Input: dimensioned drawing with shaded views. Units: mm. Origin: part minimum x, y, z. A direction names the side the tool comes from. Round coordinates to 2 decimals unless told otherwise and drop trailing zeros. Order: outer loops, then holes, each group sorted by start corner. A loop starts at its lowest first (then second) coordinate and runs counter-clockwise, first axis right, second up. Notation, with made-up numbers: (87.5, -25) - (135.5, -25) arc R18 cw to (135.5, -21) - close; hole circle Ø9 at (-9.75, 12). An arc over 180 degrees is marked (long way). Put each result on its own line as item: value. Start each with the question number.
(1) Section A-A (x = 90). Output: boundary loops of the cut face in (y, z) (1 decimal), and give its area (3 significant figures).
(2) Pull-direction query (X, two-part tool) for the marked faces 1, 2, 3 and 4; classes: released by +X, released by -X, zero draft, split by the parting line, or undercut.
(3) Section B-B (y = 33.5). Output: boundary loops of the cut face in (x, z), and give its area (3 significant figures).
(4) Material intervals for L1, parallel to X at y = 68, z = 3.5; L2, parallel to X at y = 10.5, z = 40; L3, parallel to Y at x = 12.7, z = 2 (1 decimal), sorted ascending. Write a range as [from, to].
(5) Access query for the marked faces 5, 6, 7 and 8. Directions: +Z, -Z, +X, -X, +Y, -Y. A direction counts if a zero-diameter tool reaches every point of the face in a straight line with its end or side. Return the directions, or none.
(6) Section D-D (z = 18.5). Output: boundary loops of the cut face in (x, y) (1 decimal), and give its area (3 significant figures).
(7) Section C-C (x = 12.7). Output: boundary loops of the cut face in (y, z) (1 decimal).
(8) Pin query (flat end, axial travel): P1, Ø20.5, axis at x = 95, z = 10, coming from the +Y side; P2, Ø8.5, axis at x = 50.8, y = 83.92, coming from the +Z side; P3, Ø3, axis at x = 35.5, z = 8.5, coming from the +Y side; P4, Ø20.5, axis at x = 51, y = 15.5, coming from the +Z side. Return the tip coordinate at first contact, or that it passes through.
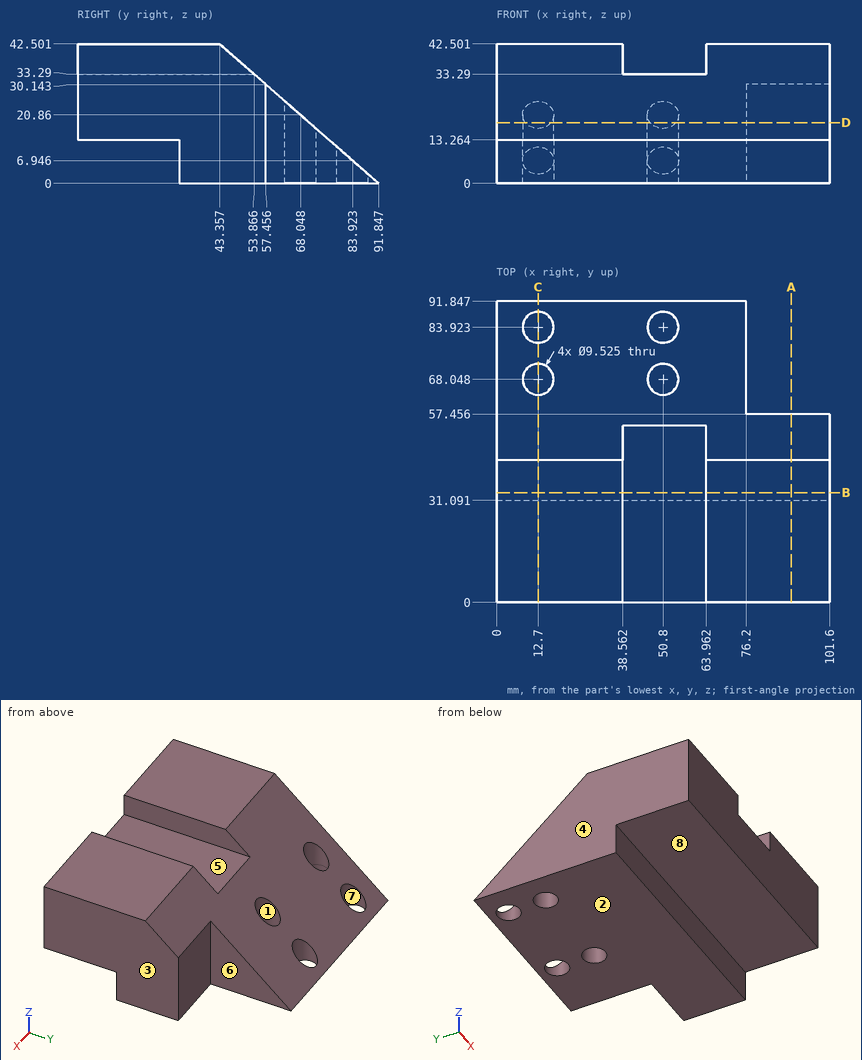
Checks:
1. outline: (0, 13.3) - (31.1, 13.3) - (31.1, 0) - (57.5, 0) - (57.5, 30.1) - (43.4, 42.5) - (0, 42.5) - close
1. area: 1,940 mm²
2. face 1: undercut
2. face 2: zero draft
2. face 3: released by +X
2. face 4: released by -X
3. outline: (0, 0) - (101.6, 0) - (101.6, 42.5) - (63.96, 42.5) - (63.96, 33.29) - (38.56, 33.29) - (38.56, 42.5) - (0, 42.5) - close
3. area: 4,080 mm²
4. L1: x = [0, 7.94], [17.46, 46.04], [55.56, 76.2]
4. L2: x = [0, 38.56], [63.96, 101.6]
4. L3: y = [31.1, 63.3], [72.8, 79.2], [88.7, 89.6]
5. face 5: +Z, +Y, -Y
5. face 6: +Z, -Z, +X, +Y
5. face 7: +Z, -Z
5. face 8: -Z, +X, -X, -Y
6. outline: (0, 0) - (101.6, 0) - (101.6, 57.5) - (76.2, 57.5) - (76.2, 70.7) - (54.7, 70.7) arc R4.8 cw (long way) to (46.9, 70.7) - (16.6, 70.7) arc R4.8 cw (long way) to (8.8, 70.7) - (0, 70.7) - close
6. area: 6,730 mm²
7. outline: (0, 13.3) - (31.1, 13.3) - (31.1, 0) - (63.3, 0) - (63.3, 25) - (43.4, 42.5) - (0, 42.5) - close; (72.8, 0) - (79.2, 0) - (79.2, 11.1) - (72.8, 16.7) - close; (88.7, 0) - (91.8, 0) - (88.7, 2.8) - close
8. P1: stops at y = 57.46
8. P2: passes through
8. P3: stops at y = 83.86
8. P4: stops at z = 33.29
